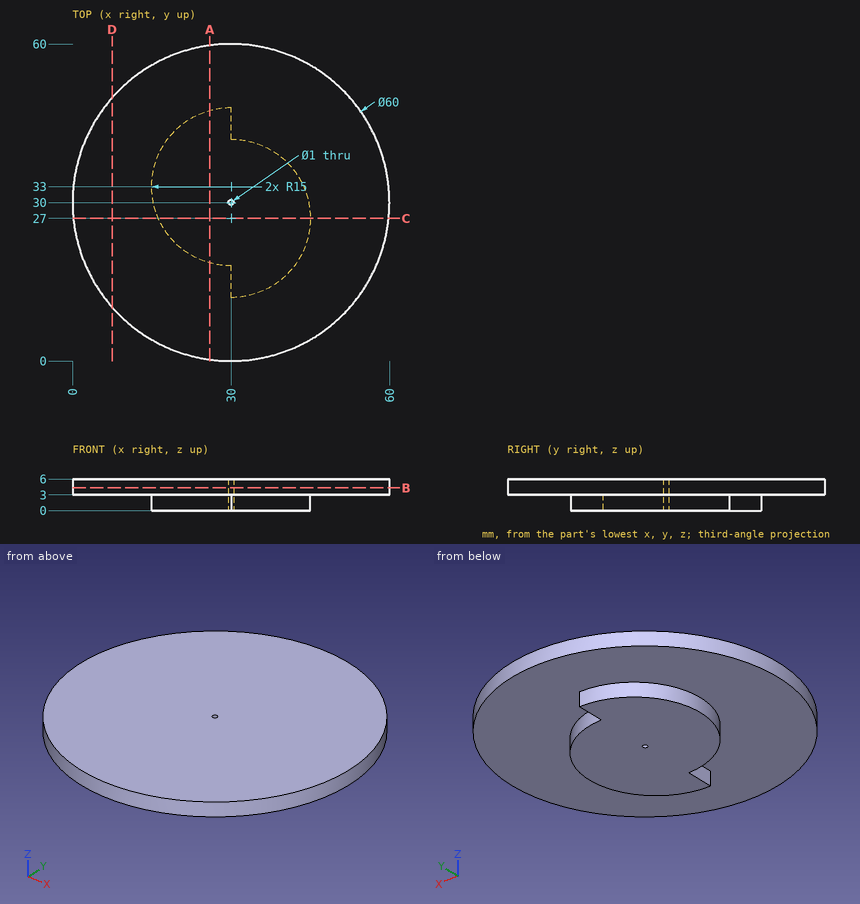
Can you work these out from the drawing? Everything is in mm from the part's minimum corner. Coordinates: 2 decimals unless noted, no trailing zeros. Loops run counter-clockwise (first coordinate to the right, second up) from the corner with the lowest first, then second, coordinate; pieces in that order, holes last. Notation, with made-up numbers: M 1.5,29 L 10.5,29 A21 ccw 10.5,41 Z; hole C 28,-28.5 d4. An arc over 180 degrees is marked long. Put each result on its own line as item: value. Start each with the question number.
(1) Will these pins go through, and if not, where does the flat tip stop? P1, Ø2, axis at x = 20.5, z = 5, coming from the -Y side; P2, Ø2.5, axis at y = 46, z = 1.5, coming from the +X side; P3, Ø2, axis at x = 10.5, z = 5, coming from the -Y side; P4, Ø3, axis at x = 47.5, z = 1, coming from the +Y side.
(2) Suppose I cut it at D-D on x = 7.5. Please give me the cut outline in (y, z).
(3) I need wall thicknesses on line 1 (Y direction, x = 30, z = 3.25); line 2 (Z direction, x = 37, y = 42); line 3 (X direction, y = 30, z = 2.4). Which ranges of each line are inside material? Lowest first, please. Write a range as from..to.
(4) Suppose I cut it at A-A on x = 26. Please give me the cut outline in (y, z), then the cut area to 3 significant figures.
(5) Suppose I cut it at C-C on y = 27. Please give me the cut outline in (x, z).
(6) Suppose I cut it at B-B on z = 4.3. Please give me the cut outline in (x, y), then the cut area to 3 significant figures.
Solutions:
1. P1: stops at y = 1.23
1. P2: stops at x = 30
1. P3: stops at y = 6.38
1. P4: passes through
2. outline: M 10.16,3 L 49.84,3 L 49.84,6 L 10.16,6 Z
3. line 1: y = 0..29.5, 30.5..60
3. line 2: z = 3..6
3. line 3: x = 15.3..29.5, 30.5..44.7
4. outline: M 0.27,3 L 18.54,3 L 18.54,0 L 47.46,0 L 47.46,3 L 59.73,3 L 59.73,6 L 0.27,6 Z
4. area: 265 mm2
5. outline: M 0.15,3 L 16.25,3 L 16.25,0 L 45,0 L 45,3 L 59.85,3 L 59.85,6 L 0.15,6 Z
6. outline: C 30,30 d60; hole C 30,30 d1
6. area: 2,830 mm2
